Geometry: final body of the model. Coordinates: model frame, mm. A direction names the side the tool comes from. Round coordinates to 2 decimals unless told otherwise and drop trailing zeros. Write each loop counter-clockwise with the first axis right and the second up, starting at its lowest first coordinate (ties: lowest second). Pieces come first, ordered by that corner, then holes. Notation, with made-up numbers: (72.5, -13.5) - (131.5, -13.5) arc R21 ccw to (131.5, 16.5) - close; hole circle Ø1 at (68, -2). An arc over 180 degrees is marked (long way). Write each question's results on one line, items separated by ' | '.
from build123d import *

# Parameters (mm, degrees)
EXTRUDE_1_DEPTH     = 5
FILLET_2_R          = 1
HOLE_WIZARD_M3_1_D  = 2.5
SKETCH_5_R          = 5
CUT_EXTRUDE_1_DEPTH = 5
HOLE_WIZARD_M12_1_D = 10.2


with BuildPart() as part:
    # 草图1 → 凸台-拉伸1 (new body)
    with BuildSketch(Plane.XY):
        Polygon((-57, 35), (-57, -35), (-12, -35), (-12, -55), (12, -55), (12, -35), (57, -35), (57, 35), (12, 35), (12, 55), (-12, 55), (-12, 35), align=None)
    extrude(amount=EXTRUDE_1_DEPTH)

    # 圆角2
    fillet_2_edges = [part.edges().sort_by_distance(p)[0] for p in [
        (-12, 55, 2.5),
        (12, 55, 2.5),
        (57, 35, 2.5),
        (57, -35, 2.5),
        (12, -55, 2.5),
        (-12, -55, 2.5),
        (-57, -35, 2.5),
        (-57, 35, 2.5),
    ]]
    fillet(fillet_2_edges, radius=FILLET_2_R)

    # M3 螺纹孔的螺纹孔钻头1 (through all)
    with Locations(Plane(origin=(-23, 9, 5), x_dir=(1, 0, 0), z_dir=(0, 0, 1))):
        with Locations((0, 0), (0, -18)):
            hole_wizard_m3_1 = Hole(HOLE_WIZARD_M3_1_D / 2)

    # 镜向1: M3 螺纹孔的螺纹孔钻头1 across plane
    add(hole_wizard_m3_1.mirror(Plane(origin=(0, 0, 0), x_dir=(0, 0, 1), z_dir=(1, 0, 0))), mode=Mode.SUBTRACT)

    # 草图5 → 切除-拉伸1 (cut)
    with BuildSketch(Plane.XY.offset(5)):
        with Locations((-48, 26)):
            Circle(SKETCH_5_R)
        with Locations((-48, -26)):
            Circle(SKETCH_5_R)
    cut_extrude_1 = extrude(amount=-CUT_EXTRUDE_1_DEPTH, mode=Mode.SUBTRACT)

    # 镜向2: 切除-拉伸1 across plane
    add(cut_extrude_1.mirror(Plane(origin=(0, 0, 0), x_dir=(0, 0, 1), z_dir=(1, 0, 0))), mode=Mode.SUBTRACT)

    # M12 螺纹孔的螺纹孔钻头1 (through all)
    with Locations(Plane(origin=(0, 47.5, 5), x_dir=(1, 0, 0), z_dir=(0, 0, 1))):
        with Locations((0, 0)):
            hole_wizard_m12_1 = Hole(HOLE_WIZARD_M12_1_D / 2)

    # 镜向3: M12 螺纹孔的螺纹孔钻头1 across plane
    add(hole_wizard_m12_1.mirror(Plane.ZX), mode=Mode.SUBTRACT)


solid = part.part
Q1. Section query B-B, the plane z = 2.75. Give the number of separate pieces and of enclosed holes in the cut face, plus the area to 3 significant figures.
Answer block:
separate pieces: 1 | enclosed holes: 10 | area: 8,440 mm2
Q2. Pin query (flat end, axial travel): pin 1 (1.5 mm diameter, centred on y = 42, z = 2, fed in from +X); pin 2 (3 mm diameter, centred on x = -41.5, z = 1, fed in from +Y); pin 3 (8 mm diameter, centred on x = 0, y = 47.5, fed in from -Z); pin 4 (1.5 mm diameter, centred on x = 29.5, z = 2.5, fed in from -Y). Return the tip coordinate at first contact, or that it passes through.
Answer block:
pin 1: x = 12 | pin 2: y = 35 | pin 3: through | pin 4: y = -35
Q3. Access query for faces 4 (the flat face through (-12, -44, 2)), 5 (the flat face through (-12, 45, 2)), 6 (the flat face through (12, 44, 2)). Directions: +Z, -Z, +X, -X, +Y, -Y. A direction counts if a zero-diameter tool reaches every point of the face in a straight line with its end or side. Return the directions, or none.
Answer block:
face 4: +Z, -Z, -X, -Y | face 5: +Z, -Z, -X, +Y | face 6: +Z, -Z, +X, +Y
Q4. Section query D-D, the plane y = -47.5. Return loops of the section in (x, z).
Answer block:
outline: (-12, 0) - (-5.1, 0) - (-5.1, 5) - (-12, 5) - close; (5.1, 0) - (12, 0) - (12, 5) - (5.1, 5) - close
Q5. Ray query, line 1 along Y through (x, z) = (48, 1.3); line 2 along Y through (x, z) = (23, 1.7); line 3 along X through (y, z) = (8.5, 1.95). Return the intervals inside material, ascending.
Answer block:
line 1: -35 to -31, -21 to 21, 31 to 35 | line 2: -35 to -10.25, -7.75 to 7.75, 10.25 to 35 | line 3: -57 to -24.15, -21.85 to 21.85, 24.15 to 57
Q6. Section query C-C, the plane x = 48. Return loops of the section in (y, z).
Answer block:
outline: (-35, 0) - (-31, 0) - (-31, 5) - (-35, 5) - close; (-21, 0) - (21, 0) - (21, 5) - (-21, 5) - close; (31, 0) - (35, 0) - (35, 5) - (31, 5) - close
Q7. Mould query, pull axis Y, two halves, no side actions, for faces 1 (the cylindrical face through (24.19, 9.38, 2.47)), 2 (the flat face through (-34, -35, 2)), 3 (the flat face through (12, -45, 2)). Classes: pulls with the +Y half, pulls with the -Y half, needs draft (parallel to the pull), parting line crosses it, or undercut.
Answer block:
face 1: undercut | face 2: pulls with the -Y half | face 3: needs draft
Q8. Section query A-A, the plane y = -26. Return loops of the section in (x, z), plus the area to 3 significant figures.
Answer block:
outline: (-57, 0) - (-53, 0) - (-53, 5) - (-57, 5) - close; (-43, 0) - (43, 0) - (43, 5) - (-43, 5) - close; (53, 0) - (57, 0) - (57, 5) - (53, 5) - close | area: 470 mm2
